from build123d import *

# Parameters (mm, degrees)
ESQUISSE1_W             = 15
ESQUISSE1_H             = 6
BOSS_EXTRU_1_DEPTH      = 10
ESQUISSE2_W             = 2
ESQUISSE2_H             = 2
ENL_V_MAT_EXTRU_1_DEPTH = 13.854960132
CONG_1_R                = 1


with BuildPart() as part:
    # Esquisse1 → Boss.-Extru.1 (new body)
    with BuildSketch(Plane.XY):
        Rectangle(ESQUISSE1_W, ESQUISSE1_H)
    extrude(amount=BOSS_EXTRU_1_DEPTH)

    # Esquisse2 → Enlèv. mat.-Extru.1 (cut, through all)
    with BuildSketch(Plane(origin=(0, 0, 0), x_dir=(-1, 0, 0), z_dir=(0, 0, -1))):
        with Locations((6.5, 2)):
            Rectangle(ESQUISSE2_W, ESQUISSE2_H)
        with Locations((6.5, -2)):
            Rectangle(ESQUISSE2_W, ESQUISSE2_H)
    extrude(amount=-ENL_V_MAT_EXTRU_1_DEPTH, mode=Mode.SUBTRACT)

    # Congé1
    cong_1_edges = [part.edges().sort_by_distance(p)[0] for p in [
        (-5.5, 1, 5),
        (-5.5, -1, 5),
    ]]
    fillet(cong_1_edges, radius=CONG_1_R)


solid = part.part
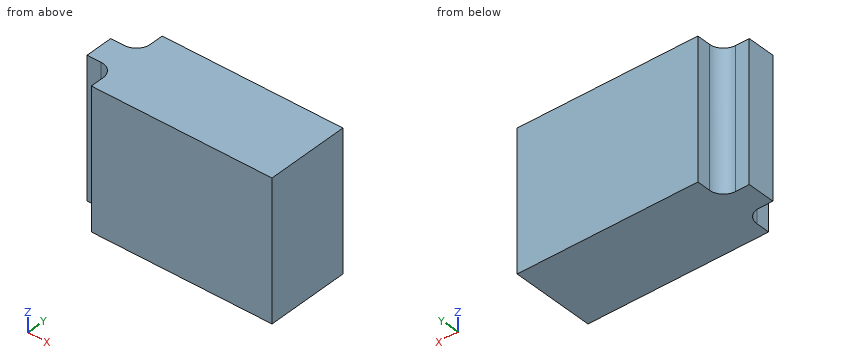
Model file for the job. Use its own axes, mm. Round coordinates to 2 decimals unless told otherwise and drop trailing zeros. Loops run counter-clockwise (first coordinate to the right, second up) from the corner with the lowest first, then second, coordinate; pieces in that order, holes last. Notation, with made-up numbers: (-5, 73) -> (42, 73) arc R22 cw to (42, 101) -> close; hole circle Ø11 at (81.25, -11). An arc over 180 degrees is marked (long way). Answer as CSV lines item,"result". Start each with the question number.
1) Slice it at C-C (y = -1.6). List the corners of the cut face in (x, z).
2) Slice it at A-A (z = 5.75). List the corners of the cut face in (x, y).
3) Pin check, flat tips, straight feed: P1, Ø0.8, axis at x = -7, z = 5.5, coming from the +Y side; P2, Ø1.1, axis at y = 2.5, z = 7, coming from the -X side. Stop position of each tip, or through.
4) Slice it at B-B (y = 2.4). List the corners of the cut face in (x, z).
5) Probe line 1 along X through (y, z) = (-2.6, 1); line 2 along Y through (x, z) = (-6, 6); line 3 along X through (y, z) = (1.2, 1.25). List the from-to ranges inside material, lowest first.
Filled in:
1,outline,"(-5.58, 0) -> (7.5, 0) -> (7.5, 10) -> (-5.58, 10) -> close"
2,outline,"(-7.5, -1) -> (-6.5, -1) arc R1 cw to (-5.5, -2) -> (-5.5, -3) -> (7.5, -3) -> (7.5, 3) -> (-5.5, 3) -> (-5.5, 2) arc R1 cw to (-6.5, 1) -> (-7.5, 1) -> close"
3,P1,"stops at y = 1"
3,P2,"stops at x = -5.5"
4,outline,"(-5.5, 0) -> (7.5, 0) -> (7.5, 10) -> (-5.5, 10) -> close"
5,line 1,"x = -5.5 to 7.5"
5,line 2,"y = -1.13 to 1.13"
5,line 3,"x = -5.9 to 7.5"
